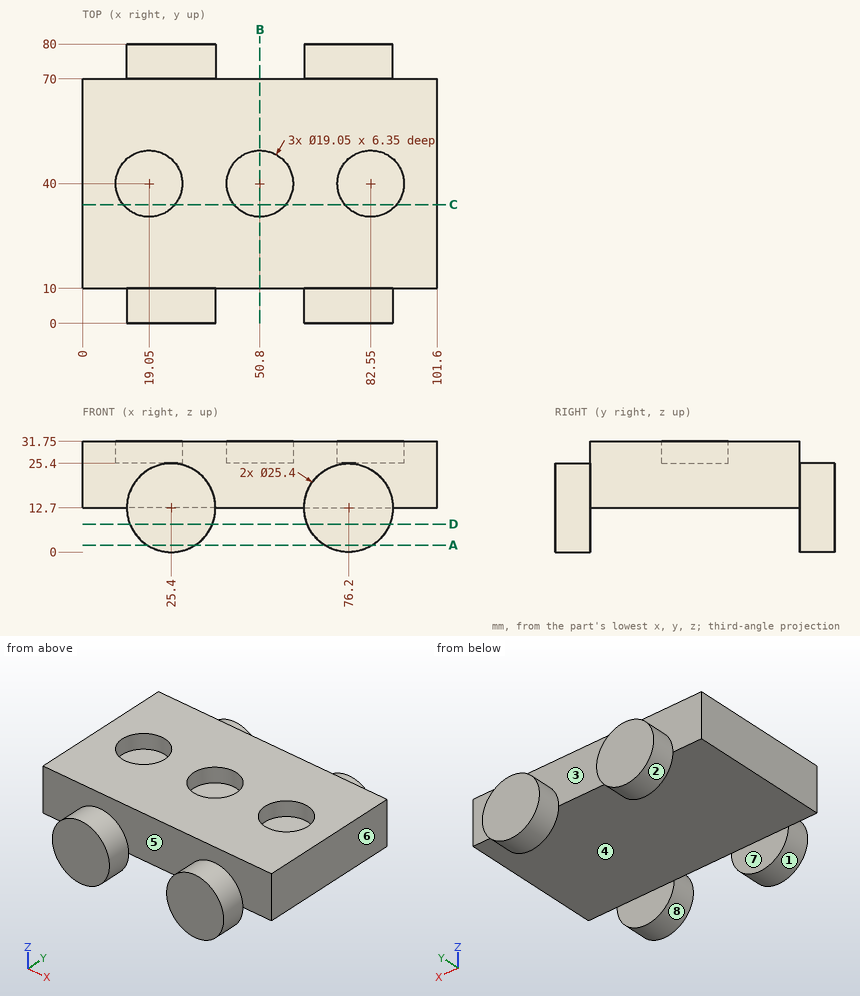
Can you work these out from the drawing? Everything is in mm from the part's minimum corner. A direction names the side the tool comes from. Coordinates: 2 decimals unless noted, no trailing zeros. Loops run counter-clockwise (first coordinate to the right, second up) from the corner with the lowest first, then second, coordinate; pieces in that order, holes last. Notation, with made-up numbers: M 13.25,32 L 67.25,32 A8 ccw 67.25,40 Z; hole C -17.75,62 d3. An arc over 180 degrees is marked long. Put each result on its own line as item: value. Start each with the question number.
(1) For the marked faces 1, 2, 3, 4 and 5, which set-ups out of +Z, -Z, +X, -X, +Y, -Y let a thin tool reach every point of the face, with its end or its side?
(2) I need wall thicknesses on line 1 (X direction, y = 40, z = 29.75) (3 decimals); line 2 (X direction, y = 8, z = 12.5); line 3 (Y direction, x = 82.55, z = 28.25) (3 decimals). Which ranges of each line are inside material? Lowest first, please. Write a range as from..to.
(3) Will these pins go through, and if not, where does the flat tip stop? P1, Ø2, axis at x = 59.5, y = 25, coming from the -Z side; P2, Ø5.5, axis at x = 17.5, y = 35.5, coming from the +Z side; P3, Ø5.5, axis at x = 37.5, z = 25.5, coming from the +Y side.
(4) Suppose I cut it at A-A on z = 2. Please give me the cut outline in (x, y).
(5) Suppose I cut it at C-C on y = 34. Please give me the cut outline in (x, z), then the cut area to 3 significant figures.
(6) Thinking about a two-plate mould opening in X: for the marked faces 6, 7 and 8, which applies, pulls with the +X half, pulls with the -X half, needs draft (parallel to the pull), parting line crosses it, or undercut?
(7) Suppose I cut it at B-B on x = 50.8. Please give me the cut outline in (y, z) (3 decimals), then the cut area to 3 significant figures.
(8) Suppose I cut it at D-D on z = 8. Please give me the cut outline in (x, y), then the cut area to 3 significant figures.
Solutions:
1. face 1: -Y
1. face 2: +Y
1. face 3: +Z, +Y
1. face 4: -Z, +X, -X
1. face 5: +Z, -Y
2. line 1: x = 0..9.525, 28.575..41.275, 60.325..73.025, 92.075..101.6
2. line 2: x = 12.7..38.1, 63.5..88.9
2. line 3: y = 10..30.475, 49.525..70
3. P1: stops at z = 12.7
3. P2: stops at z = 25.4
3. P3: stops at y = 70
4. outline: M 18.56,0 L 32.24,0 L 32.24,10 L 18.56,10 Z; M 18.56,70 L 32.24,70 L 32.24,80 L 18.56,80 Z; M 69.36,0 L 83.04,0 L 83.04,10 L 69.36,10 Z; M 69.36,70 L 83.04,70 L 83.04,80 L 69.36,80 Z
5. outline: M 0,12.7 L 101.6,12.7 L 101.6,31.75 L 89.95,31.75 L 89.95,25.4 L 75.15,25.4 L 75.15,31.75 L 58.2,31.75 L 58.2,25.4 L 43.4,25.4 L 43.4,31.75 L 26.45,31.75 L 26.45,25.4 L 11.65,25.4 L 11.65,31.75 L 0,31.75 Z
5. area: 1,650 mm2
6. face 6: pulls with the +X half
6. face 7: needs draft
6. face 8: undercut
7. outline: M 10,12.7 L 70,12.7 L 70,31.75 L 49.525,31.75 L 49.525,25.4 L 30.475,25.4 L 30.475,31.75 L 10,31.75 Z
7. area: 1,020 mm2
8. outline: M 13.6,0 L 37.2,0 L 37.2,10 L 13.6,10 Z; M 13.6,70 L 37.2,70 L 37.2,80 L 13.6,80 Z; M 64.4,0 L 88,0 L 88,10 L 64.4,10 Z; M 64.4,70 L 88,70 L 88,80 L 64.4,80 Z
8. area: 944 mm2
